```python
from build123d import *

# Parameters (mm, degrees)
ESQUISSE1_R                     = 0.75
BOSS_EXTRU_1_DEPTH              = 2.55
ESQUISSE2_R                     = 4.55
BOSS_EXTRU_2_DEPTH              = 3.55
ESQUISSE3_R                     = 3.05
ENL_V_MAT_EXTRU_1_DEPTH         = 1.5
DIAM_TRE_DU_PER_AGE_3_1_3_1_1_D = 3.1
ESQUISSE6_R                     = 2.75
ENL_V_MAT_EXTRU_2_DEPTH         = 3.5


with BuildPart() as part:
    # Esquisse1 → Boss.-Extru.1 (new body)
    with BuildSketch(Plane.XY):
        with BuildLine():
            Line((-4.500602541, 0.668637993), (-2.472858539, 14.317383513))
            ThreePointArc((-2.472858539, 14.317383513), (0, 16.45), (2.472858539, 14.317383513))
            Line((2.472858539, 14.317383513), (4.500602541, 0.668637993))
            ThreePointArc((4.500602541, 0.668637993), (0, -4.55), (-4.500602541, 0.668637993))
        make_face()
        with Locations((0, 7.725)):
            Circle(ESQUISSE1_R, mode=Mode.SUBTRACT)
        with Locations((0, 10.875)):
            Circle(ESQUISSE1_R, mode=Mode.SUBTRACT)
        with Locations((0, 14.025)):
            Circle(ESQUISSE1_R, mode=Mode.SUBTRACT)
    extrude(amount=BOSS_EXTRU_1_DEPTH)

    # Esquisse2 → Boss.-Extru.2 (add)
    with BuildSketch(Plane(origin=(0, 0, 0), x_dir=(-1, 0, 0), z_dir=(0, 0, -1))):
        Circle(ESQUISSE2_R)
    extrude(amount=BOSS_EXTRU_2_DEPTH)

    # Esquisse3 → Enlèv. mat.-Extru.1 (cut)
    with BuildSketch(Plane.XY.offset(2.55)):
        Circle(ESQUISSE3_R)
    extrude(amount=-ENL_V_MAT_EXTRU_1_DEPTH, mode=Mode.SUBTRACT)

    # Diamètre du perçage Ø3.1 (3.1)1 (through all)
    with Locations(Plane.XY.offset(1.05)):
        with Locations((0, 0)):
            Hole(DIAM_TRE_DU_PER_AGE_3_1_3_1_1_D / 2)

    # Esquisse6 → Enlèv. mat.-Extru.2 (cut)
    with BuildSketch(Plane(origin=(0, 0, -3.55), x_dir=(-1, 0, 0), z_dir=(0, 0, -1))):
        Circle(ESQUISSE6_R)
    extrude(amount=-ENL_V_MAT_EXTRU_2_DEPTH, mode=Mode.SUBTRACT)


solid = part.part
```
The listing builds one solid part. Answer for the finished solid, in the listing's coordinates (mm). A direction names the side the tool comes from. Round coordinates to 2 decimals unless told otherwise and drop trailing zeros. Order: outer loops, then holes, each group sorted by start corner. A loop starts at its lowest first (then second) coordinate and runs counter-clockwise, first axis right, second up. Notation, with made-up numbers: (47.5, 75.25) -> (87.5, 75.25) arc R11 cw to (87.5, 92.25) -> close; hole circle Ø11 at (-35, 74.5). An arc over 180 degrees is marked (long way). Answer as CSV lines item,"result". Start each with the question number.
(1) A tool of negligible diameter and unlimited length cuts with its end or side. For faces 1 (the face through (-3.047, 0.134, 1.81)), 2 (the face through (-2, 0, -0.05)), 3 (the face through (0.4, 8.36, 1.26)), from which of +Z, -Z, +X, -X, +Y, -Y can it reach the whole face along a straight path? Write none if from no direction.
(2) The part is cut by section C-C (z = -2.5). Determine the outline of the cut face in (x, y), then the cut area to 3 significant figures.
(3) For a pull along X with two mould halves and no side action, classify faces 4 (the face through (3.473, 7.589, 1.257)), 5 (the face through (-0.715, -1.375, 0.492)), 6 (the face through (0, 6, 2.55)) as +X half, -X half, draft (parallel to the pull), parting line (faces both ways), or undercut.
(4) The part is cut by section A-A (y = 0). Determine the outline of the cut face in (x, z).
(5) Find the intervals of material crossed by probe 1 along Y at (x, z) = (0, 1.8) (3 decimals); probe 2 along Y at (x, z) = (0, 0.85) (3 decimals); probe 3 along Y at (x, z) = (0, -2.1), in increasing order. Write a range as from..to.
(6) Flat-ended cylindrical pins translate along their axes: pin 1 Ø2.5 at (x, y) = (0, 0) entering from +Z; pin 2 Ø2.5 at (x, y) = (0, 10.875) entering from -Z; pin 3 Ø5 at (x, y) = (0, 0) entering from -Z. Find the tip coordinate at first contact, or state that the pin passes through.
(7) The part is cut by section D-D (z = 2). Determine the outline of the cut face in (x, y) (3 decimals), then the cut area to 3 significant figures.
(8) The part is cut by section B-B (x = 0). Count the separate pieces of the cut face and the enclosed holes in it, then the cut area to 3 significant figures.
Evaluation:
1,face 1,"+Z"
1,face 2,"-Z"
1,face 3,"+Z, -Z"
2,outline,"circle Ø9.1 at (0, 0); hole circle Ø5.5 at (0, 0)"
2,area,"41.3 mm²"
3,face 4,"+X half"
3,face 5,"undercut"
3,face 6,"draft"
4,outline,"(-4.55, -3.55) -> (-2.75, -3.55) -> (-2.75, -0.05) -> (-1.55, -0.05) -> (-1.55, 1.05) -> (-3.05, 1.05) -> (-3.05, 2.55) -> (-4.55, 2.55) -> close; (1.55, -0.05) -> (2.75, -0.05) -> (2.75, -3.55) -> (4.55, -3.55) -> (4.55, 2.55) -> (3.05, 2.55) -> (3.05, 1.05) -> (1.55, 1.05) -> close"
5,probe 1,"-4.55..-3.05, 3.05..6.975, 8.475..10.125, 11.625..13.275, 14.775..16.45"
5,probe 2,"-4.55..-1.55, 1.55..6.975, 8.475..10.125, 11.625..13.275, 14.775..16.45"
5,probe 3,"-4.55..-2.75, 2.75..4.55"
6,pin 1,"through"
6,pin 2,"z = 0"
6,pin 3,"z = -0.05"
7,outline,"(-4.501, 0.669) arc R4.55 ccw (long way) to (4.501, 0.669) -> (2.473, 14.317) arc R2.5 ccw to (-2.473, 14.317) -> close; hole circle Ø6.1 at (0, 0); hole circle Ø1.5 at (0, 7.725); hole circle Ø1.5 at (0, 10.875); hole circle Ø1.5 at (0, 14.025)"
7,area,"107 mm²"
8,separate pieces,"5"
8,enclosed holes,"0"
8,area,"42.6 mm²"
